Autodesk Inventor part; units mm, degrees
ref_plane "YZ Plane" through (0, 0, 0) normal (1, 0, 0) x (0, 1, 0)
ref_plane "XZ Plane" through (0, 0, 0) normal (0, 1, 0) x (-1, 0, 0)
ref_plane "XY Plane" through (0, 0, 0) normal (0, 0, 1) x (1, 0, 0)
sketch "Sketch1" plane through (0, 0, 0) normal (0, 1, 0) x (-1, 0, 0)
  line L0 (0, 0) -> (-188.328, 0) construction
  line L1 (0, 6) -> (-188.328, 6)
  line L2 (-188.328, -6) -> (0, -6)
  arc A0 (0, -6) -> (0, 6) centre (0, 0) ccw
  arc A1 (-188.328, 6) -> (-188.328, -6) centre (-188.328, 0) ccw
  circle A2 centre (0, 0) radius 2.1
  line L3 (-10, 0) -> (-178.328, 0) construction
  line L4 (-10, 2.1) -> (-178.328, 2.1)
  line L5 (-178.328, -2.1) -> (-10, -2.1)
  arc A3 (-10, -2.1) -> (-10, 2.1) centre (-10, 0) ccw
  arc A4 (-178.328, 2.1) -> (-178.328, -2.1) centre (-178.328, 0) ccw
  point P0 (-94.164, 0)
  point P1 (-94.164, 0)
  dimension "d0" = 188.328
  dimension "d1" = 12
  dimension "d2" = 4.2
  dimension "d3" = 4.2
  dimension "d6" = 10
  dimension "d7" = 10
extrude "Extrusion1" add sketch "Sketch1" along normal blind 5
Here's how the part is built. I have some questions about the finished solid (model axes, mm). A direction names the side the tool comes from. Give positions to 0.01 mm unless a question says otherwise; leave off trailing zeros. Loops run counter-clockwise (first coordinate to the right, second up) from the corner with the lowest first, then second, coordinate; pieces in that order, holes last. Notation, with made-up numbers: (-36.5, 50.25) -> (-8.5, 50.25) arc R33 cw to (-8.5, 81.25) -> close; hole circle Ø11 at (7.5, -37.5). An arc over 180 degrees is marked (long way). Use one line per item in the form item = value. Start each with the question number.
1) Imagine slicing it at A-A (x = 110.5). Please give me the cut outline in (y, z).
2) Please list where these lines run through material, in increasing order: line 1 along X through (y, z) = (3.25, -0.25); line 2 along Z through (x, y) = (52.5, 3.8); line 3 along X through (y, z) = (2.75, -0.75).
3) Imagine slicing it at B-B (z = 0). Please give me the cut outline in (x, y), then the cut area to 3 significant figures.
4) Thinking about a two-plate mould opening in X: for faces 1 (the face through (96, 5, 3)), 2 (the face through (-6, 2, 0)), 3 (the face through (-2.003, 2.465, -0.631)), which applies, +X half, -X half, draft (parallel to the pull), parting line (faces both ways), or undercut?
5) Which directions (+Z, -Z, +X, -X, +Y, -Y) give clear straight access to the entire face, cutting with the end or side of a thin tool? Please do faces 4 (the face through (93, 2, 6)), 5 (the face through (95, 2, -2.1)).
6) Imagine slicing it at C-C (y = 3.4). Please give me the cut outline in (x, z).
Check values:
q1.outline = (0, -6) -> (5, -6) -> (5, -2.1) -> (0, -2.1) -> close; (0, 2.1) -> (5, 2.1) -> (5, 6) -> (0, 6) -> close
q2.line_1 = -5.99 to -2.09, 2.09 to 7.91, 180.41 to 194.32
q2.line_2 = -6 to -2.1, 2.1 to 6
q2.line_3 = -5.95 to -1.96, 1.96 to 8.04, 180.29 to 194.28
q3.outline = (-6, 0) -> (-2.1, 0) -> (-2.1, 5) -> (-6, 5) -> close; (2.1, 0) -> (7.9, 0) -> (7.9, 5) -> (2.1, 5) -> close; (180.43, 0) -> (194.33, 0) -> (194.33, 5) -> (180.43, 5) -> close
q3.area = 118 mm^2
q4.face_1 = draft
q4.face_2 = -X half
q4.face_3 = undercut
q5.face_4 = +Z, +X, -X, +Y, -Y
q5.face_5 = +Y, -Y
q6.outline = (0, -6) -> (188.33, -6) arc R6 ccw to (188.33, 6) -> (0, 6) arc R6 ccw to start; hole circle Ø4.2 at (0, 0); hole (10, -2.1) -> (178.33, -2.1) arc R2.1 ccw to (178.33, 2.1) -> (10, 2.1) arc R2.1 ccw to start
